from build123d import *

# Parameters (mm, degrees)
F0_W      = 19.05
F0_H      = 19.05
F1_DEPTH  = 3.175
F2_W      = 19.05
F2_H      = 3.175
F3_DEPTH  = 15.875
F5_DEPTH  = 3.175
F7_DEPTH  = 3.175
F8_R      = 1.5875
F9_DEPTH  = 3.176
F10_R     = 1.5875
F11_DEPTH = 3.176


with BuildPart() as f1:
    # F0 (on Top) → F1 (new body)
    with BuildSketch(Plane.XY):
        Rectangle(F0_W, F0_H)
    extrude(amount=F1_DEPTH)

    # F2 (on face) → F3 (join)
    with BuildSketch(Plane(origin=(0, 0, 0), x_dir=(1, 0, 0), z_dir=(0, 0, -1))):
        with Locations((0, -7.9375)):
            Rectangle(F2_W, F2_H)
    extrude(amount=F3_DEPTH)

    # F4 (on face) → F5 (join)
    with BuildSketch(Plane(origin=(-9.525, 0, 0), x_dir=(0, -1, 0), z_dir=(-1, 0, 0))):
        Polygon((-6.35, -15.875), (9.525, 0), (-6.35, 0), align=None)
    extrude(amount=-F5_DEPTH)

    # F6 (on face) → F7 (join)
    with BuildSketch(Plane.YZ.offset(9.525)):
        Polygon((-9.525, 0), (6.35, -15.875), (6.35, 0), align=None)
    extrude(amount=-F7_DEPTH)

    # F8 (on face) → F9 (cut, through all)
    with BuildSketch(Plane.XZ.offset(-6.35)):
        with Locations((0, -7.9375)):
            Circle(F8_R)
    extrude(amount=-F9_DEPTH, mode=Mode.SUBTRACT)

    # F10 (on face) → F11 (cut, through all)
    with BuildSketch(Plane(origin=(0, 0, 0), x_dir=(1, 0, 0), z_dir=(0, 0, -1))):
        with Locations((0, 1.5875)):
            Circle(F10_R)
    extrude(amount=-F11_DEPTH, mode=Mode.SUBTRACT)


solid = f1.part
Verification items for the finished model (mm, model axes). A direction names the side the tool comes from. Coordinates: 2 decimals unless noted, no trailing zeros. Order: outer loops, then holes, each group sorted by start corner. A loop starts at its lowest first (then second) coordinate and runs counter-clockwise, first axis right, second up. Notation, with made-up numbers: (32, 68.5) -> (82, 68.5) arc R17 ccw to (82, 78.5) -> close; hole circle Ø9 at (81.25, 72). An arc over 180 degrees is marked (long way). Put each result on its own line as item: value. Start each with the question number.
1. Mould release check, pull along X, two halves, no side actions. Record for faces 1 (the flat face through (0, 9.525, -6)), 2 (the cylindrical face through (-0.21, -3.16, 1.57)), 3 (the flat face through (-9.525, 2, -4)): released by +X, released by -X, zero draft, split by the parting line, or undercut.
2. Go/stop test with a flat-tipped pin: pin 1 Ø1 at (x, y) = (3, -4) entering from -Z. Record where the tip stops, or that it passes through.
3. Cross-section at A-A, the plane x = 0. Record the boundary of the cut face in (y, z) (3 decimals).
4. Cross-section at C-C, the plane z = -12.75. Record the boundary of the cut face in (x, y) (3 decimals), then the cut area to 3 significant figures.
5. Cross-section at D-D, the plane y = 6. Record the boundary of the cut face in (x, z) (3 decimals).
6. Access from +Z, -Z, +X, -X, +Y, -Y to the whole of each face (thin tool, end or side, straight path). Record for faces 4 (the flat face through (-6.35, 0, -6)), 5 (the flat face through (9.525, 2, -4)).
7. Material ranges on L1, parallel to X at y = 5.75, z = -11.25 (3 decimals); L2, parallel to Y at x = 0, z = 1.95 (3 decimals); L3, parallel to Y at x = 6.25, z = -2 (3 decimals), recorded low to high. Write a range as [from, to].
8. Cross-section at B-B, the plane x = 3. Record the boundary of the cut face in (y, z) (3 decimals), then the cut area to 3 significant figures.
Computed:
1. face 1: zero draft
1. face 2: undercut
1. face 3: released by -X
2. pin 1: z = 0
3. outline: (-9.525, 0) -> (-3.175, 0) -> (-3.175, 3.175) -> (-9.525, 3.175) -> close; (0, 0) -> (6.35, 0) -> (6.35, -6.35) -> (9.525, -6.35) -> (9.525, 3.175) -> (0, 3.175) -> close; (6.35, -15.875) -> (9.525, -15.875) -> (9.525, -9.525) -> (6.35, -9.525) -> close
4. outline: (-9.525, 3.225) -> (-6.35, 3.225) -> (-6.35, 6.35) -> (6.35, 6.35) -> (6.35, 3.225) -> (9.525, 3.225) -> (9.525, 9.525) -> (-9.525, 9.525) -> close
4. area: 80.3 mm2
5. outline: (-9.525, -15.525) -> (-6.35, -15.525) -> (-6.35, 0) -> (6.35, 0) -> (6.35, -15.525) -> (9.525, -15.525) -> (9.525, 3.175) -> (-9.525, 3.175) -> close
6. face 4: -Z, -Y
6. face 5: +Z, -Z, +X, +Y, -Y
7. L1: [-9.525, -6.35], [6.35, 9.525]
7. L2: [-9.525, -3.175], [0, 9.525]
7. L3: [6.35, 9.525]
8. outline: (-9.525, 0) -> (6.35, 0) -> (6.35, -15.875) -> (9.525, -15.875) -> (9.525, 3.175) -> (-9.525, 3.175) -> close
8. area: 111 mm2
